Autodesk Inventor part; units mm, degrees
ref_plane "Work Plane1" through (1.0137, 23.2927, 10) normal (0, 1, 0) x (1, 0, 0)
ref_plane "YZ Plane" through (0, 0, 0) normal (1, 0, 0) x (0, 1, 0)
ref_plane "XZ Plane" through (0, 0, 0) normal (0, 1, 0) x (-1, 0, 0)
sketch "Sketch1" plane through (0, 0, 0) normal (0, 0, 1) x (1, 0, 0)
  line L0 (-18.4863, -0.9573) -> (8.5137, -0.9573)
  line L1 (8.5137, -0.9573) -> (8.5137, 2.0427)
  line L2 (8.5137, 2.0427) -> (-18.4863, 2.0427)
  line L3 (-18.4863, 2.0427) -> (-18.4863, -0.9573)
  circle A0 centre (-4.9863, 12.0427) radius 4.15
  line L4 (-4.9863, 2.0427) -> (-4.9863, 12.0427)
  line L5 (-4.9863, 12.0427) -> (-4.9863, 2.0427) construction
  line L6 (-10.9863, 12.0427) -> (-10.9863, 2.0427)
  line L7 (1.0137, 2.0427) -> (1.0137, 12.0427)
  arc A1 (1.0137, 12.0427) -> (-10.9863, 12.0427) centre (-4.9863, 12.0427) ccw
  arc A2 (-10.9863, 2.0427) -> (1.0137, 2.0427) centre (-4.9863, 2.0427) ccw
  point P0 (0, 0)
  point P1 (-4.9863, 7.0427)
  point P2 (-10.9863, 2.0427)
  dimension "d0" = 3
  dimension "d1" = 27
  dimension "d2" = 8.3
  dimension "d3" = 6
  dimension "d4" = 10
extrude "Extrusion1" add sketch "Sketch1" along normal blind 10 contours L3 L2 A2 L0 | A2 L2 L0 | A2 L2 L1 L0 | L6 A1 L7 L2
sketch "Sketch2" plane through (-18.4863, -0.9573, 0) normal (0, -1, 0) x (1, 0, 0)
  line L0 (0, 0) -> (0, 10)
  line L1 (0, 5) -> (27, 5)
  line L2 (27, 0) -> (27, 10)
  circle A0 centre (3.5, 5) radius 1.75
  line L3 (19.5, 0) -> (7.5, 0)
  line L4 (13.5, 0) -> (13.5, -6.2833)
  circle A1 centre (23.5, 5) radius 1.75
  point P0 (18.4863, 0)
  dimension "d7" = 3.5
  dimension "d8" = 20
extrude "Extrusion2" cut sketch "Sketch2" against normal up to surface (3 mm away)
fillet "Fillet1" radius 2 4 edges at (-18.4863, 0.5427, 0) (-18.4863, 0.5427, 10) (8.5137, 0.5427, 0) (8.5137, 0.5427, 10)
ref_plane "Work Plane1" through (1.0137, 23.2927, 10) normal (0, 1, 0) x (1, 0, 0)
sketch "Sketch3" plane through (1.0137, 23.2927, 10) normal (0, 1, 0) x (1, 0, 0)
  line L0 (0, 10) -> (-12, 10)
  line L1 (-12, 10) -> (-12, 0)
  line L2 (0, 0) -> (-12, 0)
  line L3 (0, 10) -> (0, 0)
  line L4 (-6, 10) -> (-6, 0)
  circle A0 centre (-6, 5) radius 1.5
  point P0 (-1.0137, 10)
  dimension "d13" = 3
extrude "Extrusion3" cut sketch "Sketch3" against normal blind 10 contours A0 L4 | L4 A0
properties part number "Rod Holder_3DPrint"
Can you work these out from the model? Positions are in its coordinate system, mm. A direction names the side the tool comes from. Round coordinates to 2 decimals unless told otherwise and drop trailing zeros. Write each loop counter-clockwise with the first axis right and the second up, starting at its lowest first coordinate (ties: lowest second). Pieces come first, ordered by that corner, then holes. Notation, with made-up numbers: M -25,52.25 L -17,52.25 A26 ccw -17,86.25 Z; hole C 10.25,-27 d2. An arc over 180 degrees is marked long. Use a Markdown table: item, result.
Item 1: We'd pull the mould along X, two halves only. Please class faces 4 (the face through (-6.092, 16.993, 3.986)), 5 (the face through (1.014, 7, 5)), 6 (the face through (-18.486, 1, 5)): released by +X, released by -X, zero draft, split by the parting line, or undercut.
Found:
| item | result |
|---|---|
| face 4 | undercut |
| face 5 | released by +X |
| face 6 | released by -X |
Item 2: If I drill on line 1 along X through (y, z) = (0.1, 5); line 2 along Z through (x, y) = (-15, 1.5); line 3 along Y through (x, z) = (1.25, 7.5), over which ranges is the centre line in solid material (lowest first)? Write a range as [from, to].
Found:
| item | result |
|---|---|
| line 1 | x = [-18.49, -16.74], [-13.24, 3.26], [6.76, 8.51] |
| line 2 | z = [0, 3.25], [6.75, 10] |
| line 3 | y = [-0.96, 2.04] |
Item 3: For pin 1 Ø2 at (y, z) = (8.5, 5.5) entering from +X; pin 2 Ø2 at (x, z) = (5, 3) entering from +Y; pin 3 Ø6 at (y, z) = (14, 6.5) entering from -X, each with a flat end and sliding along its axis, tell me the tip position at first contact or that it passes through.
Found:
| item | result |
|---|---|
| pin 1 | stops at x = 1.01 |
| pin 2 | stops at y = 2.04 |
| pin 3 | stops at x = -10.99 |
Item 4: I want a section at D-D (z = 5). List the corners of the cut face in (x, y) for me.
Found:
| item | result |
|---|---|
| outline | M -18.49,-0.96 L -16.74,-0.96 L -16.74,2.04 L -18.49,2.04 Z; M -13.24,-0.96 L 3.26,-0.96 L 3.26,2.04 L 1.01,2.04 L 1.01,12.04 A6 ccw -3.49,17.85 L -3.49,15.91 A4.15 cw long -6.49,15.91 L -6.49,17.85 A6 ccw -10.99,12.04 L -10.99,2.04 L -13.24,2.04 Z; M 6.76,-0.96 L 8.51,-0.96 L 8.51,2.04 L 6.76,2.04 Z |
Item 5: I want a section at B-B (z = 1). List the corners of the cut face in (x, y) for me.
Found:
| item | result |
|---|---|
| outline | M -18.22,-0.96 L 8.25,-0.96 L 8.25,2.04 L 1.01,2.04 L 1.01,12.04 A6 ccw -10.99,12.04 L -10.99,2.04 L -18.22,2.04 Z; hole C -4.99,12.04 d8.3 |
Item 6: Which directions (+Z, -Z, +X, -X, +Y, -Y) give clear straight access to the entire face, cutting with the end or side of a thin tool? Please do faces 1 (the face through (7.94, 0.56, 0.6)), 2 (the face through (3, 2.043, 5)), 3 (the face through (-10.986, 7, 5)).
Found:
| item | result |
|---|---|
| face 1 | -Z, +X, +Y, -Y |
| face 2 | +Z, -Z, +X, +Y |
| face 3 | +Z, -Z, -X, +Y |
Item 7: I want a section at A-A (y = 11). List the corners of the cut face in (x, z) for me.
Found:
| item | result |
|---|---|
| outline | M -10.99,0 L -9,0 L -9,10 L -10.99,10 Z; M -0.97,0 L 1.01,0 L 1.01,10 L -0.97,10 Z |
Item 8: I want a section at C-C (x = -8.25). List the corners of the cut face in (y, z) for me.
Found:
| item | result |
|---|---|
| outline | M -0.96,0 L 9.48,0 L 9.48,10 L -0.96,10 Z; M 14.61,0 L 17.08,0 L 17.08,10 L 14.61,10 Z |
